Autodesk Inventor part; units mm, degrees
ref_plane "YZ Plane" through (0, 0, 0) normal (1, 0, 0) x (0, 1, 0)
ref_plane "XZ Plane" through (0, 0, 0) normal (0, 1, 0) x (-1, 0, 0)
ref_plane "XY Plane" through (0, 0, 0) normal (0, 0, 1) x (1, 0, 0)
sketch "Sketch1" plane through (0, 0, 0) normal (0, 1, 0) x (-1, 0, 0)
  line L0 (2.55, 0.5) -> (-2.55, 0.5)
  line L1 (-2.55, 0.5) -> (-2.55, -0.5)
  line L2 (-2.55, -0.5) -> (2.55, -0.5)
  line L3 (2.55, -0.5) -> (2.55, 0.5)
  line L4 (-2.55, 0) -> (2.55, 0) construction
  point P0 (0, 0)
  point P1 (0, -0.5)
  point P2 (0, 0)
  dimension "d0" = 5.1
  dimension "d1" = 1
sketch "Sketch2" plane through (0, 0, 0) normal (0, 1, 0) x (-1, 0, 0)
  circle A0 centre (0, 0) radius 5
  dimension "d4" = 10
sketch "Sketch3" plane through (0, 0, 0) normal (0, 1, 0) x (-1, 0, 0)
  line L0 (7.5, -6) -> (-7.5, -6)
  line L1 (-7.5, -6) -> (-7.5, 6)
  line L2 (-7.5, 6) -> (7.5, 6)
  line L3 (7.5, 6) -> (7.5, -6)
  line L4 (7.5, 0) -> (-7.5, 0) construction
  line L5 (0, -6) -> (0, 6) construction
  point P0 (0, 0)
  point P1 (0, 0)
  dimension "d2" = 15
  dimension "d3" = 12
extrude "Extrusion1" add sketch "Sketch3" along normal blind 2
extrude "Extrusion2" cut sketch "Sketch1" along normal blind 2
extrude "Extrusion4" add sketch "Sketch2" along normal blind 4
sketch "Sketch7" plane through (0, 4, 0) normal (0, 1, 0) x (1, 0, 0)
  circle A0 centre (0, 0) radius 4.4878
extrude "Extrusion5" cut sketch "Sketch7" against normal blind 3
sketch "Sketch8" plane through (0, 1, 0) normal (0, 1, 0) x (1, 0, 0)
  line L0 (-2.55, 0.5) -> (2.55, 0.5)
  line L1 (2.55, 0.5) -> (2.55, -0.5)
  line L2 (2.55, -0.5) -> (-2.55, -0.5)
  line L3 (-2.55, -0.5) -> (-2.55, 0.5)
  line L4 (-2.55, 0) -> (2.55, 0) construction
  line L5 (0, 0.5) -> (0, -0.5) construction
  point P0 (0, 0)
  point P1 (0, 0)
  dimension "d15" = 5.1
  dimension "d16" = 1
extrude "Extrusion6" cut sketch "Sketch8" against normal blind 3
sketch "Sketch9" plane through (7.5, 0, -6) normal (0, 0, -1) x (-1, 0, 0)
  circle A0 centre (13.2943, 1) radius 0.75
  line L0 (7.5, 0) -> (7.5, 2) construction
  line L1 (2.5, 2) -> (12.5, 2) construction
  circle A1 centre (1.7057, 1) radius 0.75
  dimension "d19" = 1.5
extrude "Extrusion7" add sketch "Sketch9" along normal blind 20
sketch "Sketch14" plane through (5.7943, 1, -26) normal (0, 0, -1) x (-1, 0, 0)
  circle A0 centre (0, -3.14) radius 0.75
  circle A1 centre (11.5887, -3.14) radius 0.75
  circle A2 centre (11.5887, 0) radius 0.75
  line L0 (10.8387, 0) -> (10.8387, -3.14)
  line L1 (12.3387, 0) -> (12.3387, -3.14)
  circle A3 centre (0, 0) radius 0.75
  line L2 (-0.75, 0) -> (-0.75, -3.14)
  line L3 (0.75, 0) -> (0.75, -3.14)
  point P0 (5.7943, -1)
  dimension "d25" = 1.5
  dimension "d26" = 1.5
extrude "Extrusion8" add sketch "Sketch14" along normal blind 0.5
sketch "Sketch17" plane through (5.7943, 1, -26) normal (0, 0, 1) x (1, 0, 0)
  line L0 (-13.2943, -1) -> (1.7057, -1) construction
  line L1 (-0.0029, -1) -> (-0.0029, -3.1605) construction
  circle A0 centre (-0.0029, -3.1605) radius 0.6 construction
  line L2 (-5.7943, -1) -> (-5.7943, -3.1605) construction
  circle A1 centre (-0.0029, -3.1605) radius 0.6
  circle A2 centre (-11.5858, -3.1605) radius 0.6 construction
  circle A3 centre (-11.5858, -3.1605) radius 0.6
  circle A4 centre (-0.0029, -3.1605) radius 0.675
  circle A5 centre (-11.5858, -3.1605) radius 0.675
  dimension "d29" = 1.2
  dimension "d32" = 1.35
  dimension "d33" = 1.35
extrude "Extrusion9" add sketch "Sketch17" along normal blind 3 contours A1 | A3
sketch "Sketch19" plane through (5.7943, 1, -26) normal (0, 0, 1) x (1, 0, 0)
  circle A0 centre (-11.5858, -3.1605) radius 0.6
  circle A1 centre (-11.5858, -3.1605) radius 0.675
  circle A2 centre (-0.0029, -3.1605) radius 0.6
  circle A3 centre (-0.0029, -3.1605) radius 0.675
  point P0 (-5.7943, -1)
  dimension "d34" = 1.35
  dimension "d35" = 1.35
extrude "Extrusion10" add sketch "Sketch19" along normal blind 0.25
properties part number "LDR_case"
For this review, take the finished solid that the model builds, in its own axes (mm). A direction names the side the tool comes from. Give positions to 0.01 mm unless a question says otherwise; leave off trailing zeros. Write each loop counter-clockwise with the first axis right and the second up, starting at its lowest first coordinate (ties: lowest second). Pieces come first, ordered by that corner, then holes. Notation, with made-up numbers: (49.25, 80.5) -> (67.25, 80.5) arc R18 cw to (67.25, 89.5) -> close; hole circle Ø11 at (-38, -23.5). An arc over 180 degrees is marked (long way). Use CSV: the item, a comma, the result in double quotes.
Q1. Take a section at D-D, the plane z = -13. Write out the cut boundary in (x, y).
Conclusion:
outline,"circle Ø1.5 at (-5.79, 1); circle Ø1.5 at (5.79, 1)"
Q2. To check wall thickness, follow probe 1 along Z at (x, y) = (-0.5, 0.5); probe 2 along Z at (x, y) = (0, 2.6). State the ranges of each line that lie inside material, in increasing order. Write a range as [from, to].
Conclusion:
probe 1,"[-6, -0.5], [0.5, 6]"
probe 2,"[-5, -4.49], [4.49, 5]"
Q3. Tool access review of faces 4 (the face through (0, 0.5, 0.5)), 5 (the face through (0, 1, 6)), 6 (the face through (-7.5, 1, 0)), 7 (the face through (0, 1, 1)), 8 (the face through (5.192, -2.187, -24.394)): name each direction out of +Z, -Z, +X, -X, +Y, -Y from which nothing blocks a thin tool from reaching the whole face with its end or side.
Conclusion:
face 4,"+Y, -Y"
face 5,"+Z, +X, -X, +Y, -Y"
face 6,"+Z, -Z, -X, +Y, -Y"
face 7,"+Y"
face 8,"+Z"
Q4. Take a section at B-B, the plane z = 0. Write out the cut boundary in (x, y), then the cut area to 3 significant figures.
Conclusion:
outline,"(-7.5, 0) -> (-2.55, 0) -> (-2.55, 1) -> (-4.49, 1) -> (-4.49, 4) -> (-5, 4) -> (-5, 2) -> (-7.5, 2) -> close; (2.55, 0) -> (7.5, 0) -> (7.5, 2) -> (5, 2) -> (5, 4) -> (4.49, 4) -> (4.49, 1) -> (2.55, 1) -> close"
area,"18.0 mm2"
Q5. For P1, Ø3, axis at x = -1, y = 2, coming from the -Z side; P2, Ø1.5, axis at x = 0.5, z = -1.5, coming from the +Y side; P3, Ø1, axis at x = -5.5, y = -2, coming from the +Z side, all flat-tipped, find the tip position at first contact; note any pin that passes through.
Conclusion:
P1,"z = -6"
P2,"y = 1"
P3,"z = -23"
Q6. Mouldability with a two-part tool opening along X and no side actions: class faces 1 (the face through (7.5, 1, 0)), 2 (the face through (5.08, 0.77, -16.11)), 3 (the face through (-6, -2, -23)) as pulls with the +X half, pulls with the -X half, needs draft (parallel to the pull), parting line crosses it, or undercut.
Conclusion:
face 1,"pulls with the +X half"
face 2,"undercut"
face 3,"needs draft"
Q7. Take a section at A-A, the plane x = 0. Write out the cut boundary in (y, z).
Conclusion:
outline,"(0, -6) -> (2, -6) -> (2, -5) -> (4, -5) -> (4, -4.49) -> (1, -4.49) -> (1, -0.5) -> (0, -0.5) -> close; (0, 0.5) -> (1, 0.5) -> (1, 4.49) -> (4, 4.49) -> (4, 5) -> (2, 5) -> (2, 6) -> (0, 6) -> close"
Q8. Take a section at C-C, the plane y = 3. Write out the cut boundary in (x, z).
Conclusion:
outline,"circle Ø10 at (0, 0); hole circle Ø8.98 at (0, 0)"
